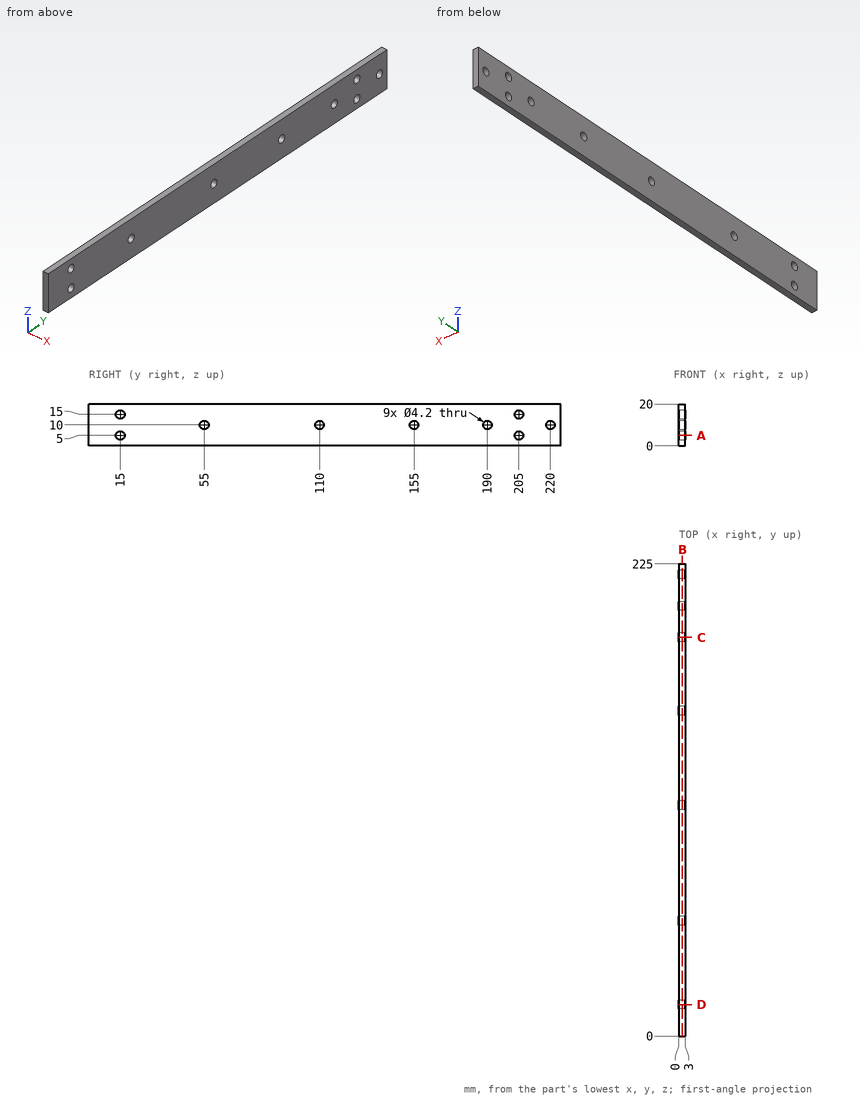
Print and shaded views of the part. All mm, measured from the part's lowest x, y and z. Round coordinates to 2 decimals unless told otherwise and drop trailing zeros. Write each loop counter-clockwise with the first axis right and the second up, starting at its lowest first coordinate (ties: lowest second). Pieces come first, ordered by that corner, then holes.
(1) Slice it at A-A, the plane z = 5. Write the cut outline in (x, y).
(2) Drop a flat-ended pin along its axis: P1, Ø2.5, axis at y = 110, z = 10, coming from the +X side. Give the stop position or say it passes through.
(3) Probe line 1 along Z through (x, y) = (1.95, 15); line 2 along Y through (x, z) = (0.9, 10); line 3 along Y through (x, z) = (1.8, 14.75). List the from-to ranges inside material, lowest first.
(4) Slice it at B-B, the plane x = 1.7. Count the separate pieces of the cut face and the enclosed holes in it, and give its area (3 significant figures).
(5) Slice it at D-D, the plane y = 15. Write the cut outline in (x, z), and give its area (3 significant figures).
(6) Slice it at C-C, the plane y = 190. Write the cut outline in (x, z), and give its area (3 significant figures).
From the geometry:
1. outline: (0, 0) - (3, 0) - (3, 12.9) - (0, 12.9) - close; (0, 17.1) - (3, 17.1) - (3, 202.9) - (0, 202.9) - close; (0, 207.1) - (3, 207.1) - (3, 225) - (0, 225) - close
2. P1: passes through
3. line 1: z = 0 to 2.9, 7.1 to 12.9, 17.1 to 20
3. line 2: y = 0 to 52.9, 57.1 to 107.9, 112.1 to 152.9, 157.1 to 187.9, 192.1 to 217.9, 222.1 to 225
3. line 3: y = 0 to 12.91, 17.09 to 202.91, 207.09 to 225
4. separate pieces: 1
4. enclosed holes: 9
4. area: 4,380 mm2
5. outline: (0, 0) - (3, 0) - (3, 2.9) - (0, 2.9) - close; (0, 7.1) - (3, 7.1) - (3, 12.9) - (0, 12.9) - close; (0, 17.1) - (3, 17.1) - (3, 20) - (0, 20) - close
5. area: 34.8 mm2
6. outline: (0, 0) - (3, 0) - (3, 7.9) - (0, 7.9) - close; (0, 12.1) - (3, 12.1) - (3, 20) - (0, 20) - close
6. area: 47.4 mm2
